The model under review builds one solid part; all positions refer to its coordinate system, in mm. A direction names the side the tool comes from. Give positions to 0.01 mm unless a question says otherwise; leave off trailing zeros. Order: outer loops, then holes, each group sorted by start corner. A loop starts at its lowest first (then second) coordinate and runs counter-clockwise, first axis right, second up.
```python
from build123d import *

# Parameters (mm, degrees)
SKETCH1_R                     = 19.05
SKETCH1_R_2                   = 2.5
BOSS_EXTRUDE1_DEPTH           = 21
SKETCH2_R                     = 1.25
CUT_EXTRUDE1_DEPTH            = 3
CUT_EXTRUDE1_DEPTH_BACK       = 15
SKETCH4_R                     = 1.25
CUT_EXTRUDE2_DEPTH            = 20
CSK_FOR_M5_SFHCS1_D           = 5.2
CSK_FOR_M5_SFHCS1_CSINK_D     = 11
CSK_FOR_M5_SFHCS1_CSINK_ANGLE = 90


with BuildPart() as part:
    # Sketch1 → Boss-Extrude1 (new body)
    with BuildSketch(Plane(origin=(0, 0, 0), x_dir=(1, 0, 0), z_dir=(0, 1, 0))):
        Circle(SKETCH1_R)
        with Locations((0, -12.525)):
            Circle(SKETCH1_R_2, mode=Mode.SUBTRACT)
        with Locations((-10.846968182, 6.2625)):
            Circle(SKETCH1_R_2, mode=Mode.SUBTRACT)
        with BuildLine():
            Line((-2, 5.656854249), (-2, 7.5))
            Line((-2, 7.5), (-1, 7.5))
            Line((-1, 7.5), (1, 7.5))
            Line((1, 7.5), (2, 7.5))
            Line((2, 7.5), (2, 5.656854249))
            ThreePointArc((2, 5.656854249), (4.898979486, 3.464101615), (6, 0))
            ThreePointArc((6, 0), (-3.464101615, -4.898979486), (-2, 5.656854249))
        make_face(mode=Mode.SUBTRACT)
        with Locations((10.846968182, 6.2625)):
            Circle(SKETCH1_R_2, mode=Mode.SUBTRACT)
        with Locations((-10.846968182, 6.2625)):
            Circle(SKETCH1_R_2)
        with Locations((10.846968182, 6.2625)):
            Circle(SKETCH1_R_2)
        with Locations((0, -12.525)):
            Circle(SKETCH1_R_2)
    extrude(amount=BOSS_EXTRUDE1_DEPTH)

    # Sketch2 → Cut-Extrude1 (cut, two sides)
    with BuildSketch(Plane.XY.offset(-7.5)) as cut_extrude1_sk:
        with Locations((0, 18)):
            Circle(SKETCH2_R)
    extrude(amount=CUT_EXTRUDE1_DEPTH, mode=Mode.SUBTRACT)
    extrude(cut_extrude1_sk.sketch, amount=-CUT_EXTRUDE1_DEPTH_BACK, mode=Mode.SUBTRACT)

    # Sketch4 → Cut-Extrude2 (cut)
    with BuildSketch(Plane(origin=(0, 0, 0), x_dir=(0, -1, 0), z_dir=(-0.866025404, 0, 0.5))):
        with Locations((-18, 0)):
            Circle(SKETCH4_R)
    extrude(amount=CUT_EXTRUDE2_DEPTH, mode=Mode.SUBTRACT)

    # CSK for M5 SFHCS1 (through all)
    with Locations(Plane(origin=(0, 21, 0), x_dir=(1, 0, 0), z_dir=(0, 1, 0))):
        with Locations((10.846968182, 6.2625), (0, -12.525), (-10.846968182, 6.2625), (0, 0)):
            CounterSinkHole(CSK_FOR_M5_SFHCS1_D / 2, CSK_FOR_M5_SFHCS1_CSINK_D / 2, counter_sink_angle=CSK_FOR_M5_SFHCS1_CSINK_ANGLE)


solid = part.part
```
Item 1: Take a section at B-B (y = 8). Give the number of separate pieces and of enclosed holes in the cut face, and give its area (3 significant figures).
Values found:
separate pieces: 1
enclosed holes: 4
area: 957 mm2
Item 2: Take a section at C-C (z = -13). Give the boundary of the cut face in (x, y).
Values found:
outline: (-13.92, 0) - (13.92, 0) - (13.92, 21) - (-13.92, 21) - close; hole circle Ø2.5 at (0, 18)
Item 3: Clearance check with flat-ended pins moving along their axes: pin 1 Ø6 at (x, z) = (-9, 2.5) entering from -Y; pin 2 Ø5 at (x, y) = (-4, 12.5) entering from -Z; pin 3 Ø12 at (y, z) = (17.5, -8) entering from +X; pin 4 Ø6 at (x, y) = (14.5, 6) entering from -Z. State where each tip first meets the part, or that it passes through.
Values found:
pin 1: stops at y = 0
pin 2: stops at z = -18.99
pin 3: stops at x = 18.94
pin 4: stops at z = -15.19
Item 4: Draft analysis for pull direction X (two halves, no side actions). For faces 1 (the flat face through (2, 10, -7)), 2 (the flat face through (-5, 0, -5)), 3 (the conical face through (0.59, 18.24, 15.2)), 4 (the cylindrical face through (-15.12, 10.35, 11.59)), state which applies: released by +X, released by -X, zero draft, split by the parting line, or undercut.
Values found:
face 1: undercut
face 2: zero draft
face 3: undercut
face 4: split by the parting line
Item 5: For line 1 (Z direction, x = 0, y = 14.5) (3 decimals); line 2 (Y direction, x = 0, z = -12); line 3 (X direction, y = 6.5, z = -5), list the stretches that pass through material, from the lowest coordinate up.
Values found:
line 1: z = -19.05 to -7.5, 6 to 9.925, 15.125 to 19.05
line 2: y = 0 to 16.75, 19.25 to 21
line 3: x = -18.38 to -13.12, -8.57 to -3.32, 3.32 to 8.57, 13.12 to 18.38
Item 6: For faces 5 (the cylindrical face through (-0.27, 16.78, -13.19)), 6 (the flat face through (-5, 21, -5)), 7 (the flat face through (-2, 10, -7)), list the 3-axis set-ups (+Z, -Z, +X, -X, +Y, -Y) from which the entire face can be reached by the end or side of a thin tool; tool diameter is ignored.
Values found:
face 5: -Z
face 6: +Z, -Z, +X, -X, +Y
face 7: +Y, -Y
Item 7: Take a section at A-A (x = 0). Give the boundary of the cut face in (y, z) (3 decimals).
Values found:
outline: (0, -19.05) - (16.75, -19.05) - (16.75, -7.5) - (0, -7.5) - close; (0, 6) - (21, 6) - (21, 7.025) - (18.1, 9.925) - (0, 9.925) - close; (0, 15.125) - (18.1, 15.125) - (21, 18.025) - (21, 19.05) - (0, 19.05) - close; (19.25, -19.05) - (21, -19.05) - (21, -7.5) - (19.25, -7.5) - close
